Geometry check sheet. Reference: the model listing, model coordinates, mm. A direction names the side the tool comes from. Round coordinates to 2 decimals unless told otherwise and drop trailing zeros. Order: outer loops, then holes, each group sorted by start corner. A loop starts at its lowest first (then second) coordinate and runs counter-clockwise, first axis right, second up.
```python
from build123d import *

# Parameters (mm, degrees)
F1_DEPTH = 10


with BuildPart() as f1:
    # F0 (on Front) → F1 (new body)
    with BuildSketch(Plane.XZ):
        with BuildLine():
            Line((0, 14), (0, 0))
            Line((0, 0), (5, 0))
            ThreePointArc((5, 0), (10.117275, 1.408522), (13.792991, 5.237301))
            ThreePointArc((13.792991, 5.237301), (20.570263, 11.429803), (29.726646, 12.092483))
            Line((29.726646, 12.092483), (45, 8))
            Line((45, 8), (60, 8))
            Line((60, 8), (65, 13))
            Line((65, 13), (65, 17))
            Line((65, 17), (52.349352, 17))
            ThreePointArc((52.349352, 17), (46.736865, 18.089572), (41.939741, 21.2))
            ThreePointArc((41.939741, 21.2), (38.741657, 23.273618), (35, 24))
            Line((35, 24), (10, 24))
            Line((10, 24), (0, 14))
        make_face()
    extrude(amount=F1_DEPTH)


solid = f1.part
```
(1) Sectioned sample at B-B, the plane y = -2.5. Record the cut outline in (x, z).
Returned:
outline: (0, 0) - (5, 0) arc R10 ccw to (13.79, 5.24) arc R14 cw to (29.73, 12.09) - (45, 8) - (60, 8) - (65, 13) - (65, 17) - (52.35, 17) arc R15 cw to (41.94, 21.2) arc R10 ccw to (35, 24) - (10, 24) - (0, 14) - close
(2) Set-up check for faces 5 (the flat face through (52, -5, 8)), 6 (the flat face through (37.256, -4.93, 10.075)), 7 (the flat face through (59, -5, 17)), 8 (the flat face through (5, -5, 19)): record each of +Z, -Z, +X, -X, +Y, -Y from which the full face is reachable in a straight line by a thin tool's end or side.
Returned:
face 5: -Z, +X, +Y, -Y
face 6: -Z, +Y, -Y
face 7: +Z, +X, +Y, -Y
face 8: +Z, -X, +Y, -Y
(3) Sectioned sample at C-C, the plane x = 14.5. Record the cut outline in (y, z), and give its area (3 significant figures).
Returned:
outline: (-10, 6.4) - (0, 6.4) - (0, 24) - (-10, 24) - close
area: 176 mm2
(4) Material ranges on line 1 (Z direction, x = 59, y = -1.5); line 2 (Z direction, x = 26.5, y = -7.5); line 3 (X direction, y = -9, z = 15), recorded low to high.
Returned:
line 1: z = 8 to 17
line 2: z = 12.56 to 24
line 3: x = 1 to 65
(5) Sectioned sample at D-D, the plane x = 25. Record the cut outline in (y, z).
Returned:
outline: (-10, 12.53) - (0, 12.53) - (0, 24) - (-10, 24) - close
(6) Sectioned sample at A-A, the plane z = 10.5. Record the cut outline in (x, y), and give its area (3 significant figures).
Returned:
outline: (0, -10) - (18.78, -10) - (18.78, 0) - (0, 0) - close; (35.67, -10) - (62.5, -10) - (62.5, 0) - (35.67, 0) - close
area: 456 mm2
(7) Draft check along X on faces 1 (the flat face through (0, -5, 7)), 2 (the cylindrical face through (10.1, -4.9, 1.4)), 3 (the flat face through (25, -10, 15)), 4 (the cylindrical face through (20.5, -4.9, 11.4)). Enter one of: released by +X, released by -X, zero draft, split by the parting line, or undercut.
Returned:
face 1: released by -X
face 2: released by +X
face 3: zero draft
face 4: undercut
(8) Depth check by flat-ended pin: P1, Ø4, axis at x = 23.5, y = -2.5, coming from the -Z side; P2, Ø6, axis at x = 55, y = -6.5, coming from the -Z side; P3, Ø3, axis at y = -2, z = 7.5, coming from the +X side. Enter the tip coordinate at first touch or a pass-through.
Returned:
P1: stops at z = 11.79
P2: stops at z = 8
P3: stops at x = 61
